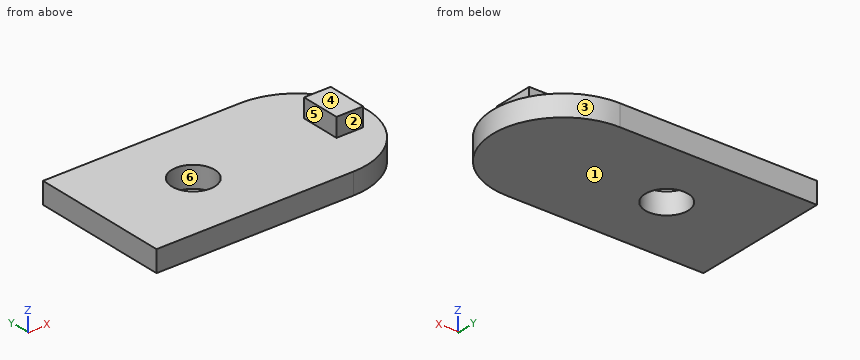
Autodesk Inventor part; units mm, degrees
ref_plane "YZ Plane" through (0, 0, 0) normal (1, 0, 0) x (0, 1, 0)
ref_plane "XZ Plane" through (0, 0, 0) normal (0, 1, 0) x (-1, 0, 0)
ref_plane "XY Plane" through (0, 0, 0) normal (0, 0, 1) x (1, 0, 0)
sketch "Sketch1" plane through (0, 0, 0) normal (0, 0, 1) x (1, 0, 0)
  line L0 (0, 0) -> (14.75, 0)
  arc A0 (14.75, 0) -> (14.75, 10.5) centre (14.75, 5.25) ccw
  line L1 (14.75, 10.5) -> (0, 10.5)
  line L2 (0, 10.5) -> (0, 0)
  dimension "d0" = 10.5
  dimension "d1" = 20
extrude "Extrusion1" add sketch "Sketch1" along normal blind 1.6
sketch "Esquisse2" plane through (0, 0, 1.6) normal (0, 0, 1) x (1, 0, 0)
  line L0 (0, 0) -> (14.75, 0) construction
  arc A0 (14.75, 0) -> (14.75, 10.5) centre (14.75, 5.25) ccw construction
  line L1 (14.75, 10.5) -> (0, 10.5) construction
  line L2 (0, 10.5) -> (0, 0) construction
  line L3 (16.5, 6.75) -> (18.5, 6.75)
  line L4 (18.5, 6.75) -> (18.5, 3.75)
  line L5 (18.5, 3.75) -> (16.5, 3.75)
  line L6 (16.5, 3.75) -> (16.5, 6.75)
  point P0 (16.5, 5.25)
  dimension "d4" = 3
  dimension "d5" = 2
  dimension "d6" = 18.5
extrude "Extrusion2" add sketch "Esquisse2" along normal blind 1.4
sketch "Esquisse3" plane through (0, 0, 1.6) normal (0, 0, 1) x (1, 0, 0)
  line L0 (18.5, 6.75) -> (18.5, 3.75) construction
  line L1 (18.5, 3.75) -> (16.5, 3.75) construction
  line L2 (16.5, 3.75) -> (16.5, 6.75) construction
  line L3 (16.5, 6.75) -> (18.5, 6.75) construction
  line L4 (0, 0) -> (14.75, 0) construction
  arc A0 (14.75, 0) -> (14.75, 10.5) centre (14.75, 5.25) ccw construction
  line L5 (14.75, 10.5) -> (0, 10.5) construction
  line L6 (0, 10.5) -> (0, 0) construction
  line L7 (0, 5.25) -> (14.75, 5.25) construction
  point P0 (7, 5.25)
  dimension "d9" = 7
hole "Perçage1" at (7, 5.25, 1.6) direction (0, 0, -1) diameter 3.2 end through all
properties part number "FE015" material "Fourniture / Geliefertes"
The listing builds one solid part. Answer for the finished solid, in the listing's coordinates (mm). Face numbers are marked on the shaded views. A direction names the side the tool comes from. Give positions to 0.01 mm unless a question says otherwise; leave off trailing zeros. Write each loop counter-clockwise with the first axis right and the second up, starting at its lowest first coordinate (ties: lowest second). Pieces come first, ordered by that corner, then holes.
Item 1: Section C-C, the plane x = 7 is taken. Write down the section's boundary in (y, z).
Item 2: Which of the six approach directions +Z, -Z, +X, -X, +Y, -Y give full straight-line access (tool end or side, diameter ignored) to the marked faces 1 and 2?
Item 3: Section D-D, the plane x = 5 is taken. Write down the section's boundary in (y, z).
Item 4: Section A-A, the plane z = 0.9 is taken. Write down the section's boundary in (x, y).
Item 5: Determine the mould class of the marked faces 3, 4, 5 and 6 for opening direction X: released by +X, released by -X, zero draft, split by the parting line, or undercut.
Item 6: Flat-ended cylindrical pins translate along their axes: P1, Ø1.1, axis at y = 6, z = 2.5, coming from the +X side; P2, Ø1.9, axis at x = 7, y = 5.25, coming from the -Z side; P3, Ø0.7, axis at x = 17, z = 2.5, coming from the +Y side; P4, Ø5, axis at x = 5, y = 7.5, coming from the +Z side. Find the tip coordinate at first contact, or state that the pin passes through.
Item 7: Find the intervals of material crossed by line 1 along X through (y, z) = (5.25, 0.95); line 2 along Y through (x, z) = (7, 1.35); line 3 along Z through (x, y) = (14.5, 6), in increasing order.
Item 8: Section B-B, the plane y = 5.25 is taken. Write down the section's boundary in (x, z).
Completed:
1. outline: (0, 0) - (3.65, 0) - (3.65, 1.6) - (0, 1.6) - close; (6.85, 0) - (10.5, 0) - (10.5, 1.6) - (6.85, 1.6) - close
2. face 1: -Z, +X, -X, +Y, -Y
2. face 2: +Z, +X, -X, -Y
3. outline: (0, 0) - (10.5, 0) - (10.5, 1.6) - (0, 1.6) - close
4. outline: (0, 0) - (14.75, 0) arc R5.25 ccw to (14.75, 10.5) - (0, 10.5) - close; hole circle Ø3.2 at (7, 5.25)
5. face 3: released by +X
5. face 4: zero draft
5. face 5: released by -X
5. face 6: undercut
6. P1: stops at x = 18.5
6. P2: passes through
6. P3: stops at y = 6.75
6. P4: stops at z = 1.6
7. line 1: x = 0 to 5.4, 8.6 to 20
7. line 2: y = 0 to 3.65, 6.85 to 10.5
7. line 3: z = 0 to 1.6
8. outline: (0, 0) - (5.4, 0) - (5.4, 1.6) - (0, 1.6) - close; (8.6, 0) - (20, 0) - (20, 1.6) - (18.5, 1.6) - (18.5, 3) - (16.5, 3) - (16.5, 1.6) - (8.6, 1.6) - close
